Autodesk Inventor part; units mm, degrees
ref_plane "YZ Plane" through (0, 0, 0) normal (1, 0, 0) x (0, 1, 0)
ref_plane "XZ Plane" through (0, 0, 0) normal (0, 1, 0) x (-1, 0, 0)
ref_plane "XY Plane" through (0, 0, 0) normal (0, 0, 1) x (1, 0, 0)
sketch "Boceto1" plane through (0, 0, 0) normal (0, 1, 0) x (-1, 0, 0)
  arc A0 (-10.02, 7.27) -> (-8.75, 6) centre (-8.75, 7.27) ccw
  line L0 (-8.75, 6) -> (-2.54, 6)
  arc A1 (-1.27, 4.73) -> (-2.54, 6) centre (-2.54, 4.73) ccw
  line L1 (-1.27, 4.73) -> (-1.27, 1.27)
  arc A2 (-1.27, 1.27) -> (0, 0) centre (0, 1.27) ccw
  line L2 (0, 0) -> (62.46, 0)
  arc A3 (62.46, 0) -> (63.73, 1.27) centre (62.46, 1.27) ccw
  line L3 (63.73, 1.27) -> (63.73, 4.73)
  arc A4 (65, 6) -> (63.73, 4.73) centre (65, 4.73) ccw
  line L4 (65, 6) -> (71.21, 6)
  arc A5 (71.21, 6) -> (72.48, 7.27) centre (71.21, 7.27) ccw
  line L5 (72.48, 7.27) -> (72.48, 21.73)
  arc A6 (72.48, 21.73) -> (71.21, 23) centre (71.21, 21.73) ccw
  line L6 (71.21, 23) -> (65, 23)
  arc A7 (63.73, 24.27) -> (65, 23) centre (65, 24.27) ccw
  line L7 (63.73, 24.27) -> (63.73, 27.73)
  arc A8 (63.73, 27.73) -> (62.46, 29) centre (62.46, 27.73) ccw
  line L8 (62.46, 29) -> (0, 29)
  arc A9 (0, 29) -> (-1.27, 27.73) centre (0, 27.73) ccw
  line L9 (-1.27, 27.73) -> (-1.27, 24.27)
  arc A10 (-2.54, 23) -> (-1.27, 24.27) centre (-2.54, 24.27) ccw
  line L10 (-2.54, 23) -> (-8.75, 23)
  arc A11 (-8.75, 23) -> (-10.02, 21.73) centre (-8.75, 21.73) ccw
  line L11 (-10.02, 21.73) -> (-10.02, 7.27)
  circle A12 centre (55.955, 14.5) radius 7.4
  circle A13 centre (61.755, 25.475) radius 1.25
  circle A14 centre (0.755, 3.475) radius 1.25
  circle A15 centre (0.755, 25.475) radius 1.25
  circle A16 centre (61.755, 3.475) radius 1.25
  circle A17 centre (38.73, 14.5) radius 0.9
  circle A18 centre (23.73, 14.5) radius 0.9
  point P0 (0, 0)
extrude "Extrusión1" add sketch "Boceto1" along normal blind 1.04
sketch "Boceto2" plane through (0, 1.04, 0) normal (0, 1, 0) x (1, 0, 0)
  circle A0 centre (3.02, -14.5) radius 0.9
  line L0 (-71.21, -23) -> (-65, -23)
  line L1 (-72.48, -7.27) -> (-72.48, -21.73)
  line L2 (2.54, -23) -> (8.75, -23)
  line L3 (10.02, -21.73) -> (10.02, -7.27)
  point P0 (0, 0)
  dimension "d3" = 1.8
  dimension "d6" = 8.5
  dimension "d7" = 7
hole "Agujero1" at (3.02, 1.04, 14.5) direction (0, -1, 0) diameter 1.8 end through all
sketch "Boceto3" plane through (0, 0, 0) normal (0, -1, 0) x (1, 0, 0)
  circle A0 centre (-3.08, 17.04) radius 0.4
  line L0 (10.02, 21.73) -> (10.02, 7.27)
  line L1 (-62.46, 29) -> (0, 29)
  circle A1 centre (-3.08, 14.5) radius 0.4
  circle A2 centre (-3.08, 11.96) radius 0.4
  line L2 (0, 0) -> (-62.46, 0)
  dimension "d15" = 0.8
  dimension "d16" = 13.1
  dimension "d17" = 11.96
  dimension "d18" = 0.8
  dimension "d19" = 0.8
  dimension "d20" = 13.1
  dimension "d21" = 13.1
  dimension "d22" = 11.96
  dimension "d23" = 2.54
  dimension "d24" = 2.54
hole "Agujero2" at (-3.08, 0, 17.04) at (-3.08, 0, 14.5) at (-3.08, 0, 11.96) direction (0, 1, 0) diameter 0.8 end through all
sketch "Boceto4" plane through (0, 1.04, 0) normal (0, 1, 0) x (1, 0, 0)
  line L0 (4.72, -19.4) -> (1.32, -19.4)
  line L1 (1.32, -19.4) -> (1.32, -17)
  line L2 (1.32, -17) -> (4.72, -17)
  line L3 (4.72, -17) -> (4.72, -19.4)
  line L4 (2.54, -23) -> (8.75, -23)
  line L5 (10.02, -21.73) -> (10.02, -7.27)
  line L6 (4.72, -12) -> (1.32, -12)
  line L7 (1.32, -12) -> (1.32, -9.6)
  line L8 (1.32, -9.6) -> (4.72, -9.6)
  line L9 (4.72, -9.6) -> (4.72, -12)
  line L10 (8.75, -6) -> (2.54, -6)
  point P0 (0, 0)
  dimension "d32" = 3.4
  dimension "d33" = 2.4
  dimension "d34" = 3.6
  dimension "d35" = 5.3
  dimension "d36" = 2.4
  dimension "d37" = 5.3
  dimension "d38" = 3.6
extrude "Extrusión2" cut sketch "Boceto4" against normal through all
properties part number "Interstage B2"
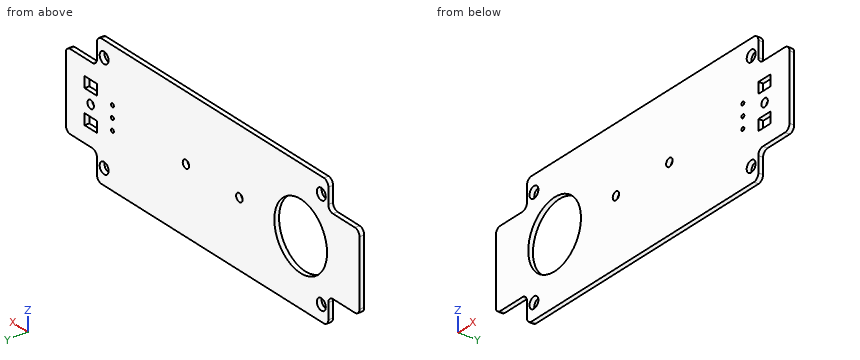
The model under review builds one solid part; all positions refer to its coordinate system, in mm. Round coordinates to 2 decimals unless told otherwise and drop trailing zeros. Loops run counter-clockwise (first coordinate to the right, second up) from the corner with the lowest first, then second, coordinate; pieces in that order, holes last. Notation, with made-up numbers: M -23.5,23 L -16.5,23 A13 cw -16.5,47 Z; hole C 39.25,-14.75 d8. An arc over 180 degrees is marked long. Answer as a JSON object with one key per item and string values.
(1) Clearance check with flat-ended pins moving along their axes: P1, Ø10, axis at x = -62.5, z = 20.5, coming from the -Y side; P2, Ø0.5, axis at x = 2, y = 0.5, coming from the +Z side. State where each tip first meets the part, or that it passes through.
Resolved:
{"P1": "y = 0", "P2": "z = 23.28"}
(2) Take a section at A-A on x = -38.73. Give the boundary of the cut face in (y, z), and give its area (3 significant figures).
Resolved:
{"outline": "M 0,0 L 1.04,0 L 1.04,13.6 L 0,13.6 Z; M 0,15.4 L 1.04,15.4 L 1.04,29 L 0,29 Z", "area": "28.3 mm²"}
(3) To check wall thickness, follow line 1 along Z through (x, y) = (4.5, 0.2); line 2 along Z through (x, y) = (-3.08, 0.45); line 3 along X through (y, z) = (0.2, 15). State the ranges of each line that lie inside material, in increasing order.
Resolved:
{"line 1": "6 to 9.6, 12 to 17, 19.4 to 23", "line 2": "0 to 11.56, 12.36 to 14.1, 14.9 to 16.64, 17.44 to 29", "line 3": "-72.48 to -63.34, -48.57 to -39.48, -37.98 to -24.48, -22.98 to 2.27, 3.77 to 10.02"}
(4) Take a section at B-B on z = 8.75. Give the boundary of the cut face in (x, y), and give its area (3 significant figures).
Resolved:
{"outline": "M -72.48,0 L -60.61,0 L -60.61,1.04 L -72.48,1.04 Z; M -51.3,0 L 10.02,0 L 10.02,1.04 L -51.3,1.04 Z", "area": "76.1 mm²"}
(5) Take a section at C-C on y = 0.5. Count the separate pieces of the cut face and the enclosed holes in it, and give its area (3 significant figures).
Resolved:
{"separate pieces": "1", "enclosed holes": "13", "area": "1,960 mm²"}
